Can you work these out from the model? Positions are in its coordinate system, mm. Give positions to 0.01 mm unless a question says otherwise; leave off trailing zeros. Write each loop counter-clockwise with the first axis right and the second up, starting at its lowest first coordinate (ties: lowest second). Pieces come first, ordered by that corner, then holes.
1. Thinking about a two-plate mould opening in Y: for faces 1 (the flat face through (6, 16.51, -6)), 2 (the flat face through (-15.2, 16.51, -10)), 3 (the cylindrical face through (-25.4, 8.14, -0.15)), which applies, pulls with the +Y half, pulls with the -Y half, needs draft (parallel to the pull), parting line crosses it, or undercut?
2. Suppose I cut it at A-A (y = 15.25). Please give me the cut outline in (x, z).
3. Suppose I cut it at C-C (y = 7.75). Please give me the cut outline in (x, z), and give its area (3 significant figures).
4. Suppose I cut it at D-D (y = 22.25). Please give me the cut outline in (x, z).
5. If I drill on probe 1 along Y at (x, z) = (-9, -7.5); probe 2 along Y at (x, z) = (1, -6.5); probe 3 along X at (y, z) = (15, 12), over which ranges is the centre line in solid material (lowest first)?
6. I'm going to push flat-ended pins straight in: pin 1 (8 mm diameter, centred on x = 11, z = -12, fed in from +Y); pin 2 (1 mm diameter, centred on x = 14, z = 5, fed in from +Y); pin 3 (12 mm diameter, centred on x = -13.5, z = -9.5, fed in from +Y). Where does each tip first touch, or does it pass through?
7. Suppose I cut it at B-B (x = -19.05). Please give me the cut outline in (y, z), and give its area (3 significant figures).
```python
from build123d import *

# Parameters (mm, degrees)
SKETCH1_R           = 19.05
BOSS_EXTRUDE1_DEPTH = 16.51


with BuildPart() as part:
    # Sketch1 → Boss-Extrude1 (new body)
    with BuildSketch(Plane(origin=(0, 0, 0), x_dir=(1, 0, 0), z_dir=(0, 1, 0))):
        Circle(SKETCH1_R)
        with BuildLine():
            ThreePointArc((-17.991666667, -6.261184437), (-19.05, 0), (-17.991666667, 6.261184437))
            ThreePointArc((-17.991666667, 6.261184437), (-25.4, 0), (-17.991666667, -6.261184437))
        make_face()
        with BuildLine():
            ThreePointArc((17.991666667, 6.261184437), (18.783553311, 3.175), (19.05, 0))
            ThreePointArc((19.05, 0), (18.783553311, -3.175), (17.991666667, -6.261184437))
            ThreePointArc((17.991666667, -6.261184437), (25.4, 0), (17.991666667, 6.261184437))
        make_face()
    extrude(amount=BOSS_EXTRUDE1_DEPTH)

    # Sketch2 → Cut-Revolve4 (revolve, cut)
    with BuildSketch(Plane(origin=(0, 16.51, 0), x_dir=(1, 0, 0), z_dir=(0, 1, 0))):
        with BuildLine():
            Line((7.62, 0), (0, 0))
            Line((0, 0), (-7.62, 0))
            ThreePointArc((-7.62, 0), (0, -7.62), (7.62, 0))
        make_face()
        with BuildLine():
            Line((13.335, 0), (7.62, 0))
            ThreePointArc((7.62, 0), (0, -7.62), (-7.62, 0))
            Line((-7.62, 0), (-13.335, 0))
            ThreePointArc((-13.335, 0), (0, -13.335), (13.335, 0))
        make_face()
    revolve(axis=Axis((0, 16.51, 0), (1, 0, 0)), mode=Mode.SUBTRACT)



with BuildPart() as body_2:
    # Sketch2_7 → Revolve1 (revolve)
    with BuildSketch(Plane(origin=(0, 16.51, 0), x_dir=(1, 0, 0), z_dir=(0, 1, 0))):
        with BuildLine():
            Line((7.62, 0), (0, 0))
            Line((0, 0), (-7.62, 0))
            ThreePointArc((-7.62, 0), (0, -7.62), (7.62, 0))
        make_face()
    revolve(axis=Axis((0, 16.51, 0), (1, 0, 0)))


with BuildPart() as part_1:
    add(part.part)

    add(body_2.part)  # Revolve2 merges body 2
    # Sketch3 → Revolve2 (revolve)
    with BuildSketch(Plane.XY, mode=Mode.PRIVATE) as revolve2_sk:
        with BuildLine():
            Line((-17.991666667, 16.51), (-7.62, 16.51))
            add(Edge.make_bspline(
                [(-6.225616872, 20.903870112), (-7.600669831, 18.930780111), (-7.62, 16.51)],
                knots=[0, 0, 0, 1, 1, 1], degree=2))
            add(Edge.make_bspline(
                [(-17.991666667, 16.51), (-13.949922169, 17.401477486), (-9.562250003, 18.24582827), (-6.225616872, 20.903870112)],
                knots=[0, 0, 0, 0, 1, 1, 1, 1], degree=3))
        make_face()
    revolve(revolve2_sk.sketch.rotate(Axis((0, 16.51, 0), (0, 1, 0)), 270), axis=Axis((0, 16.51, 0), (0, 1, 0)))


solid = part_1.part
```
Checks:
1. face 1: undercut
1. face 2: pulls with the +Y half
1. face 3: needs draft
2. outline: (-17.99, -6.26) arc R19.05 ccw to (17.99, -6.26) arc R6.35 ccw (long way) to (17.99, 6.26) arc R19.05 ccw to (-17.99, 6.26) arc R6.35 ccw (long way) to start; circle Ø15.03 at (0, 0); hole circle Ø26.55 at (0, 0)
3. outline: (-17.99, -6.26) arc R19.05 ccw to (17.99, -6.26) arc R6.35 ccw (long way) to (17.99, 6.26) arc R19.05 ccw to (-17.99, 6.26) arc R6.35 ccw (long way) to start; hole circle Ø20.11 at (0, 0)
3. area: 958 mm2
4. outline: circle Ø10.02 at (0, 0)
5. probe 1: y = 0 to 10.14, 16.51 to 18.09
5. probe 2: y = 0 to 4.91, 12.66 to 20.63
5. probe 3: x = -14.8 to -5.62, 5.62 to 14.8
6. pin 1: stops at y = 17.91
6. pin 2: stops at y = 17.33
6. pin 3: stops at y = 18.52
7. outline: (0, -6.35) - (16.51, -6.35) - (16.51, 6.35) - (0, 6.35) - close
7. area: 210 mm2
